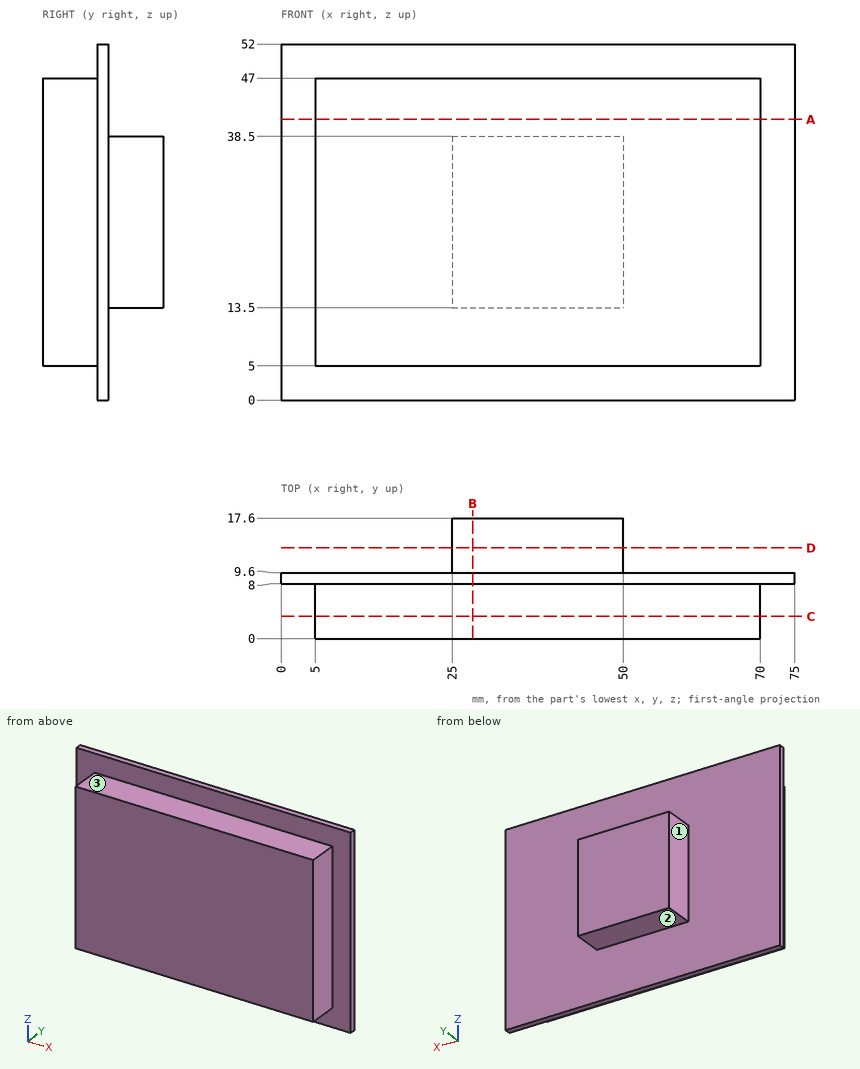
Geometry: see drawing. Coordinates: mm, zero at the bounding-box minimum. A direction names the side the tool comes from. Give positions to 0.01 mm unless a question says otherwise; leave off trailing zeros. Write each loop counter-clockwise with the first axis right and the second up, starting at its lowest first coordinate (ties: lowest second). Pieces come first, ordered by that corner, then holes. Notation, with made-up numbers: M -25,20.5 L -11,20.5 A20 cw -11,55.5 Z; hole C 51,-28 d10. An arc over 180 degrees is marked long. Answer as a JSON object with one key per item and string values.
Q1. Contact query for flat-ended pins moving along their axis: P1, Ø4, axis at x = 50.5, y = 4, coming from the -Z side; P2, Ø6.5, axis at x = 32.5, y = 13.5, coming from the -Z side; P3, Ø4, axis at y = 5, z = 27, coming from the +X side. Output: stop coordinate, or through.
Geometry check:
{"P1": "stops at z = 5", "P2": "stops at z = 13.5", "P3": "stops at x = 70"}
Q2. Access query for the marked faces 1, 2 and 3. Directions: +Z, -Z, +X, -X, +Y, -Y. A direction counts if a zero-diameter tool reaches every point of the face in a straight line with its end or side. Return the directions, or none.
Geometry check:
{"face 1": "+Z, -Z, -X, +Y", "face 2": "-Z, +X, -X, +Y", "face 3": "+Z, +X, -X, -Y"}
Q3. Cut plane B-B, the plane x = 28. Return the cut outline in (y, z).
Geometry check:
{"outline": "M 0,5 L 8,5 L 8,0 L 9.6,0 L 9.6,13.5 L 17.6,13.5 L 17.6,38.5 L 9.6,38.5 L 9.6,52 L 8,52 L 8,47 L 0,47 Z"}
Q4. Ray query, line 1 along Y through (x, z) = (12, 29); line 2 along Y through (x, z) = (71, 29.5); line 3 along Z through (x, y) = (46, 3.25). Return the intervals inside material, ascending.
Geometry check:
{"line 1": "y = 0 to 9.6", "line 2": "y = 8 to 9.6", "line 3": "z = 5 to 47"}
Q5. Cut plane C-C, the plane y = 3.25. Return the cut outline in (x, z), then the cut area to 3 significant figures.
Geometry check:
{"outline": "M 5,5 L 70,5 L 70,47 L 5,47 Z", "area": "2,730 mm^2"}
Q6. Cut plane D-D, the plane y = 13.25. Return the cut outline in (x, z).
Geometry check:
{"outline": "M 25,13.5 L 50,13.5 L 50,38.5 L 25,38.5 Z"}
Q7. Cut plane A-A, the plane z = 41. Return the cut outline in (x, y), then the cut area to 3 significant figures.
Geometry check:
{"outline": "M 0,8 L 5,8 L 5,0 L 70,0 L 70,8 L 75,8 L 75,9.6 L 0,9.6 Z", "area": "640 mm^2"}
